Autodesk Inventor part; units mm, degrees
ref_plane "YZ Plane" through (0, 0, 0) normal (1, 0, 0) x (0, 1, 0)
ref_plane "XZ Plane" through (0, 0, 0) normal (0, 1, 0) x (-1, 0, 0)
ref_plane "XY Plane" through (0, 0, 0) normal (0, 0, 1) x (1, 0, 0)
sketch "Sketch1" plane through (0, 0, 0) normal (0, 1, 0) x (-1, 0, 0)
  line L0 (13.796, 28.5881) -> (3.796, 28.5881)
  line L1 (1.796, 26.5881) -> (1.796, -29.4119)
  line L2 (3.796, -31.4119) -> (13.796, -31.4119)
  line L3 (15.796, -29.4119) -> (15.796, 26.5881)
  arc A0 (15.796, 26.5881) -> (13.796, 28.5881) centre (13.796, 26.5881) ccw
  arc A1 (13.796, -31.4119) -> (15.796, -29.4119) centre (13.796, -29.4119) ccw
  arc A2 (1.796, -29.4119) -> (3.796, -31.4119) centre (3.796, -29.4119) ccw
  arc A3 (3.796, 28.5881) -> (1.796, 26.5881) centre (3.796, 26.5881) ccw
  line L4 (14.196, 28.9881) -> (3.396, 28.9881)
  line L5 (1.396, 26.9881) -> (1.396, -29.8119)
  line L6 (3.396, -31.8119) -> (14.196, -31.8119)
  line L7 (16.196, -29.8119) -> (16.196, 26.9881)
  arc A4 (16.196, 26.9881) -> (14.196, 28.9881) centre (14.196, 26.9881) ccw
  arc A5 (14.196, -31.8119) -> (16.196, -29.8119) centre (14.196, -29.8119) ccw
  arc A6 (1.396, -29.8119) -> (3.396, -31.8119) centre (3.396, -29.8119) ccw
  arc A7 (3.396, 28.9881) -> (1.396, 26.9881) centre (3.396, 26.9881) ccw
  point P0 (0, 0)
  point P1 (15.796, 28.5881)
  point P2 (1.796, -31.4119)
  point P3 (15.796, -31.4119)
  dimension "d0" = 60
  dimension "d1" = 14
  dimension "d2" = 2
  dimension "d3" = 0.4
  dimension "d4" = 0.4
  dimension "d5" = 0.4
  dimension "d6" = 0.4
  dimension "d7" = 2
extrude "Extrusion1" add sketch "Sketch1" along normal blind 20
properties part number "cinta"
Work out the finished part from the listing and answer in its coordinate system (mm). A direction names the side the tool comes from. Round coordinates to 2 decimals unless told otherwise and drop trailing zeros. Write each loop counter-clockwise with the first axis right and the second up, starting at its lowest first coordinate (ties: lowest second). Pieces come first, ordered by that corner, then holes. Notation, with made-up numbers: (84, 83) -> (97, 83) arc R17 cw to (97, 115) -> close; hole circle Ø1 at (33.25, -6.75). An arc over 180 degrees is marked (long way). Write each question's results on one line, items separated by ' | '.
Item 1: A flat-ended cylindrical pin translates along its axis: P1, Ø8, axis at x = -7.5, z = -20.5, coming from the +Y side. Find the tip coordinate at first contact, or state that the pin passes through.
Result set:
P1: through
Item 2: A cutting plane is placed at C-C, the plane y = 2. Determine the outline of the cut face in (x, z).
Result set:
outline: (-16.2, -29.81) arc R2 ccw to (-14.2, -31.81) -> (-3.4, -31.81) arc R2 ccw to (-1.4, -29.81) -> (-1.4, 26.99) arc R2 ccw to (-3.4, 28.99) -> (-14.2, 28.99) arc R2 ccw to (-16.2, 26.99) -> close; hole (-15.8, -29.41) arc R2 ccw to (-13.8, -31.41) -> (-3.8, -31.41) arc R2 ccw to (-1.8, -29.41) -> (-1.8, 26.59) arc R2 ccw to (-3.8, 28.59) -> (-13.8, 28.59) arc R2 ccw to (-15.8, 26.59) -> close
Item 3: Find the intervals of material crossed by line 1 along X through (y, z) = (11.25, 1.5); line 2 along Z through (x, y) = (-6, 7.25); line 3 along Z through (x, y) = (-15.25, 9), in increasing order. Write a range as [from, to].
Result set:
line 1: [-16.2, -15.8], [-1.8, -1.4] | line 2: [-31.81, -31.41], [28.59, 28.99] | line 3: [-31.51, -30.79], [27.96, 28.69]
Item 4: The mould has two halves that part along Z. Classify faces 3 (the face through (-1.396, 10, -1)), 4 (the face through (-1.796, 10, -1)), 5 (the face through (-15.796, 10, -2)), 6 (the face through (-9, 10, 28.988)): +Z half, -Z half, draft (parallel to the pull), parting line (faces both ways), or undercut.
Result set:
face 3: draft | face 4: undercut | face 5: undercut | face 6: +Z half
Item 5: A cutting plane is placed at A-A, the plane x = -9.5. Determine the outline of the cut face in (y, z).
Result set:
outline: (0, -31.81) -> (20, -31.81) -> (20, -31.41) -> (0, -31.41) -> close; (0, 28.59) -> (20, 28.59) -> (20, 28.99) -> (0, 28.99) -> close
Item 6: Which of the six approach directions +Z, -Z, +X, -X, +Y, -Y give full straight-line access (tool end or side, diameter ignored) to faces 1 (the face through (-9, 10, 28.588)), 2 (the face through (-16, 20, -1))?
Result set:
face 1: +Y, -Y | face 2: +Z, -Z, +X, -X, +Y
Item 7: A cutting plane is placed at B-B, the plane z = -27. Determine the outline of the cut face in (x, y).
Result set:
outline: (-16.2, 0) -> (-15.8, 0) -> (-15.8, 20) -> (-16.2, 20) -> close; (-1.8, 0) -> (-1.4, 0) -> (-1.4, 20) -> (-1.8, 20) -> close
